```python
from build123d import *

# Parameters (mm, degrees)
SKETCH1_W           = 1.016
SKETCH1_H           = 14.732
SKETCH1_W_2         = 7.14375
SKETCH1_H_2         = 1.016
SKETCH1_W_3         = 3.945946328
SKETCH1_H_3         = 0.762
SKETCH2_R           = 6.12775
BOSS_EXTRUDE1_DEPTH = 10.16


with BuildPart() as part:
    # Sketch1 → Revolve1 (revolve)
    with BuildSketch(Plane(origin=(0, 0, 0), x_dir=(1, 0, 0), z_dir=(0, 1, 0))):
        with Locations((6.63575, 5.334)):
            Rectangle(SKETCH1_W, SKETCH1_H)
        with Locations((3.571875, 13.208)):
            Rectangle(SKETCH1_W_2, SKETCH1_H_2)
        with Locations((1.972973164, 14.097)):
            Rectangle(SKETCH1_W_3, SKETCH1_H_3)
    revolve(axis=Axis((0, 0, 288.756429932), (0, 0, -1)))

    # Sketch2 → Boss-Extrude1 (add)
    with BuildSketch(Plane.XY):
        Polygon((8.248891971, 0), (4.124445986, 7.14375), (-4.124445986, 7.14375), (-8.248891971, 0), (-4.124445986, -7.14375), (4.124445986, -7.14375), align=None)
        Circle(SKETCH2_R, mode=Mode.SUBTRACT)
    extrude(amount=-BOSS_EXTRUDE1_DEPTH)


solid = part.part
```
Geometry check sheet. Reference: the model listing, model coordinates, mm. A direction names the side the tool comes from. Round coordinates to 2 decimals unless told otherwise and drop trailing zeros. Order: outer loops, then holes, each group sorted by start corner. A loop starts at its lowest first (then second) coordinate and runs counter-clockwise, first axis right, second up. Notation, with made-up numbers: (15.5, 46) - (29.5, 46) arc R24 ccw to (29.5, 74) - close; hole circle Ø4 at (4.5, 44). An arc over 180 degrees is marked (long way). Use a Markdown table: item, result. Add a question column.
1) Gauge pin test, flat ends, axial feed: P1, Ø6, axis at x = 2.5, y = -1.5, coming from the +Z side; P2, Ø3, axis at x = 3, y = -5.5, coming from the -Z side; P3, Ø1, axis at x = 1, z = -11.5, coming from the -Y side. Record the tip position at first contact, or that the pin passes through.
2) Section check A-A (z = -7.5). Record the cut outline in (x, y), then the cut area to 3 significant figures.
3) Section check C-C (y = 5). Record the cut outline in (x, z).
4) Section check B-B (x = 3.25). Record the cut outline in (y, z).
5) Mould release check, pull along X, two halves, no side actions. Record for faces 6 (the flat face through (0, 0, -12.7)), 7 (the flat face through (6.216, 3.522, -5.009)), 8 (the flat face through (7.4, 0, 0)): released by +X, released by -X, zero draft, split by the parting line, or undercut.
6) Set-up check for faces 1 (the cylindrical face through (-7.137, -0.314, 1.002)), 2 (the flat face through (3.8, -6.4, 0)), 3 (the flat face through (-3.6, -6.4, 0)), 4 (the flat face through (3.8, 6.4, 0)), 5 (the flat face through (-3, 3, -13.716)): record each of +Z, -Z, +X, -X, +Y, -Y from which the full face is reachable in a straight line by a thin tool's end or side.
7) Thickness scan on line 1 along Z through (x, y) = (-3.75, -3.75); line 2 along Y through (x, z) = (2, -2); line 3 along Y through (x, z) = (0, -2.75). Record the ranges inside material, lowest first.
8) Section check D-D (z = 0.5). Record the cut outline in (x, y).
Established:
| question | item | result |
|---|---|---|
| 1 | P1 | z = -12.7 |
| 1 | P2 | z = -13.72 |
| 1 | P3 | y = -7.13 |
| 2 | outline | (-8.25, 0) - (-4.12, -7.14) - (4.12, -7.14) - (8.25, 0) - (4.12, 7.14) - (-4.12, 7.14) - close; hole circle Ø12.26 at (0, 0) |
| 2 | area | 58.8 mm2 |
| 3 | outline | (-5.36, -10.16) - (-5.1, -10.16) - (-5.1, -13.72) - (5.1, -13.72) - (5.1, -10.16) - (5.36, -10.16) - (5.36, 0) - (5.1, 0) - (5.1, 2.03) - (3.54, 2.03) - (3.54, -12.7) - (-3.54, -12.7) - (-3.54, 2.03) - (-5.1, 2.03) - (-5.1, 0) - (-5.36, 0) - close |
| 4 | outline | (-7.14, -10.16) - (-6.36, -10.16) - (-6.36, -13.72) - (-2.24, -13.72) - (-2.24, -14.48) - (2.24, -14.48) - (2.24, -13.72) - (6.36, -13.72) - (6.36, -10.16) - (7.14, -10.16) - (7.14, 0) - (6.36, 0) - (6.36, 2.03) - (5.19, 2.03) - (5.19, -12.7) - (-5.19, -12.7) - (-5.19, 2.03) - (-6.36, 2.03) - (-6.36, 0) - (-7.14, 0) - close |
| 5 | face 6 | undercut |
| 5 | face 7 | released by +X |
| 5 | face 8 | zero draft |
| 6 | face 1 | +Z |
| 6 | face 2 | +Z, +X, -Y |
| 6 | face 3 | +Z, -X, -Y |
| 6 | face 4 | +Z, +X, +Y |
| 6 | face 5 | -Z |
| 7 | line 1 | -13.72 to -12.7 |
| 7 | line 2 | -7.14 to -5.79, 5.79 to 7.14 |
| 7 | line 3 | -7.14 to -6.13, 6.13 to 7.14 |
| 8 | outline | circle Ø14.29 at (0, 0); hole circle Ø12.26 at (0, 0) |
